Geometry check sheet. Reference: the model listing, model coordinates, mm. A direction names the side the tool comes from. Give positions to 0.01 mm unless a question says otherwise; leave off trailing zeros. Write each loop counter-clockwise with the first axis right and the second up, starting at its lowest first coordinate (ties: lowest second). Pieces come first, ordered by that corner, then holes.
(1) Thickness scan on line 1 along Z through (x, y) = (-1.75, -3.5); line 2 along Y through (x, z) = (-2, 1); line 3 along Y through (x, z) = (0, 1.5). Record the ranges inside material, lowest first.
(2) Tool access check on faces 1 (the flat face through (3.3, -2.2, 1.46)), 2 (the flat face through (-2, -5, 1.588)), 3 (the flat face through (3.3, -2.2, -1.46)). Record the directions out of +Z, -Z, +X, -X, +Y, -Y that give a thin tool (end or side, any length) a straight path to the whole face; none if there is none.
(3) Cross-section at C-C (z = 1.25). Record the boundary of the cut face in (x, y), and give its area (3 significant figures).
```python
from build123d import *

# Parameters (mm, degrees)
SKETCH1_R             = 6.35
SKETCH1_R_2           = 5.08
BOSS_EXTRUDE1_DEPTH   = 1.5875
SKETCH1_R_3           = 3.652012
SKETCH1_R_4           = 2.382012
BOSS_EXTRUDE1_2_DEPTH = 1.5875
SKETCH2_R             = 5.08
SKETCH2_R_2           = 3.652012
BOSS_EXTRUDE2_DEPTH   = 1.4605
FILLET1_R             = 0.127
CHAMFER1_SIZE         = 0.127


with BuildPart() as part:
    # Sketch1 → Boss-Extrude1 (new, symmetric)
    with BuildSketch(Plane.XY):
        Circle(SKETCH1_R)
        Circle(SKETCH1_R_2, mode=Mode.SUBTRACT)
    extrude(amount=BOSS_EXTRUDE1_DEPTH, both=True)



with BuildPart() as body_2:
    # Sketch1 → Boss-Extrude1 2 (new, symmetric)
    with BuildSketch(Plane.XY):
        Circle(SKETCH1_R_3)
        Circle(SKETCH1_R_4, mode=Mode.SUBTRACT)
    extrude(amount=BOSS_EXTRUDE1_2_DEPTH, both=True)


with BuildPart() as part_1:
    add(part.part)

    add(body_2.part)  # Boss-Extrude2 merges body 2
    # Sketch2 → Boss-Extrude2 (add, symmetric)
    with BuildSketch(Plane.XY):
        Circle(SKETCH2_R)
        Circle(SKETCH2_R_2, mode=Mode.SUBTRACT)
    extrude(amount=BOSS_EXTRUDE2_DEPTH, both=True)

    # Fillet1
    fillet1_edges = [part_1.edges().sort_by_distance(p)[0] for p in [
        (-6.35, 0, 1.5875),
        (-6.35, 0, -1.5875),
    ]]
    fillet(fillet1_edges, radius=FILLET1_R)

    # Chamfer1
    chamfer1_edges = [part_1.edges().sort_by_distance(p)[0] for p in [
        (-2.382012, 0, 1.5875),
        (-2.382012, 0, -1.5875),
    ]]
    chamfer(chamfer1_edges, length=CHAMFER1_SIZE)


solid = part_1.part
```
Reply:
1. line 1: z = -1.46 to 1.46
1. line 2: y = -6.03 to -1.29, 1.29 to 6.03
1. line 3: y = -6.34 to -5.08, -3.65 to -2.42, 2.42 to 3.65, 5.08 to 6.34
2. face 1: +Z
2. face 2: +Z, +X, -X, +Y, -Y
2. face 3: -Z
3. outline: circle Ø12.7 at (0, 0); hole circle Ø4.76 at (0, 0)
3. area: 109 mm2
